For this review, use the dimensioned drawing (mm, ordinates from the lowest corner) and the shaded views. Coordinates: 2 decimals unless noted, no trailing zeros. Order: outer loops, then holes, each group sorted by start corner. A loop starts at its lowest first (then second) coordinate and runs counter-clockwise, first axis right, second up. Notation, with made-up numbers: (-11.5, 76.25) -> (24.5, 76.25) arc R24 ccw to (24.5, 113.25) -> close; hole circle Ø2 at (17.5, -35). An arc over 180 degrees is marked (long way). Use one line per item in the form item = value. Start each with the question number.
(1) Mouldability with a two-part tool opening along Z and no side actions: class the marked faces 1, 2 and 3 as +Z half, -Z half, draft (parallel to the pull), parting line (faces both ways), or undercut.
(2) Insertion check: pin 1 Ø1 at (x, z) = (18.5, 7.5) entering from +Y; pin 2 Ø6 at (x, z) = (19.5, 10.5) entering from -Y; pin 3 Ø1.8 at (x, z) = (21, 11.5) entering from -Y. Each pin has a flat end and moves straight along its axis. Give the tip position at first contact, or say it passes through.
(3) Take a section at D-D (z = 18.25). State the section outline as (x, y) points, then the cut area to 3 significant figures.
(4) Take a section at C-C (x = 14.75). State the section outline as (y, z) points, then the cut area to 3 significant figures.
(5) Wall thickness on line 1 along Z through (x, y) = (11.5, 0.75); line 2 along Y through (x, z) = (4, 19); line 3 along X through (y, z) = (0.9, 3.25): over which ranges is each line inside the solid? List them lowest first.
(6) Take a section at A-A (x = 11.5). State the section outline as (y, z) points.
(7) Take a section at B-B (z = 11.5). State the section outline as (x, y) points, then the cut area to 3 significant figures.
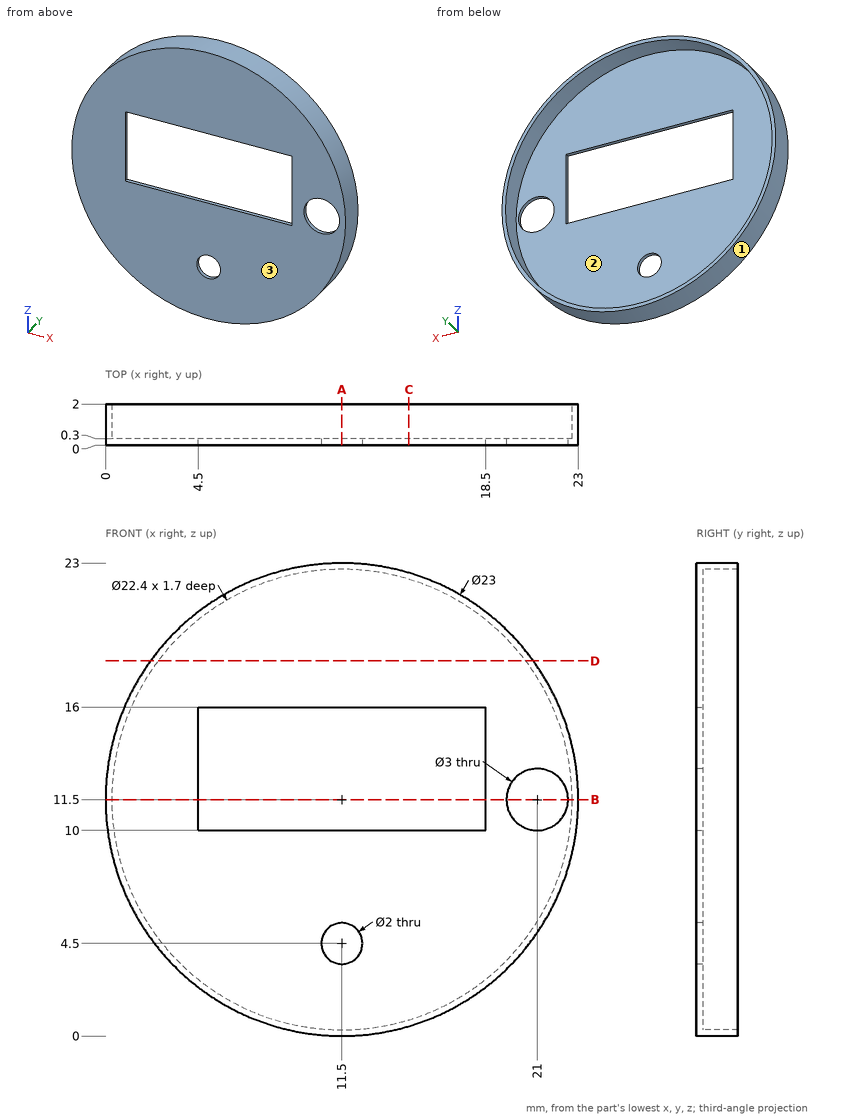
Findings:
q1.face_1 = parting line
q1.face_2 = undercut
q1.face_3 = draft
q2.pin_1 = 0.3
q2.pin_2 = 0
q2.pin_3 = through
q3.outline = (2.19, 0) -> (20.81, 0) -> (20.81, 2) -> (20.44, 2) -> (20.44, 0.3) -> (2.56, 0.3) -> (2.56, 2) -> (2.19, 2) -> close
q3.area = 6.86 mm²
q4.outline = (0, 0.47) -> (2, 0.47) -> (2, 0.78) -> (0.3, 0.78) -> (0.3, 10) -> (0, 10) -> close; (0, 16) -> (0.3, 16) -> (0.3, 22.22) -> (2, 22.22) -> (2, 22.53) -> (0, 22.53) -> close
q4.area = 5.88 mm²
q5.line_1 = 0 to 0.3, 22.7 to 23
q5.line_2 = 0 to 0.3
q5.line_3 = 3.49 to 3.93, 19.07 to 19.51
q6.outline = (0, 0) -> (2, 0) -> (2, 0.3) -> (0.3, 0.3) -> (0.3, 3.5) -> (0, 3.5) -> close; (0, 5.5) -> (0.3, 5.5) -> (0.3, 10) -> (0, 10) -> close; (0, 16) -> (0.3, 16) -> (0.3, 22.7) -> (2, 22.7) -> (2, 23) -> (0, 23) -> close
q7.outline = (0, 0) -> (4.5, 0) -> (4.5, 0.3) -> (0.3, 0.3) -> (0.3, 2) -> (0, 2) -> close; (18.5, 0) -> (19.5, 0) -> (19.5, 0.3) -> (18.5, 0.3) -> close; (22.5, 0) -> (23, 0) -> (23, 2) -> (22.7, 2) -> (22.7, 0.3) -> (22.5, 0.3) -> close
q7.area = 2.82 mm²
